Autodesk Inventor part; units mm, degrees
ref_plane "YZ Plane" through (0, 0, 0) normal (1, 0, 0) x (0, 1, 0)
ref_plane "XZ Plane" through (0, 0, 0) normal (0, 1, 0) x (-1, 0, 0)
ref_plane "XY Plane" through (0, 0, 0) normal (0, 0, 1) x (1, 0, 0)
sketch "Sketch1" plane through (0, 0, 0) normal (0, 0, 1) x (1, 0, 0)
  circle A0 centre (0, 0) radius 1.5
  circle A1 centre (0, 0) radius 3.5
  circle A2 centre (0, 0) radius 5.75 construction
  line L0 (0, 0) -> (0, 5.75) construction
  circle A3 centre (0.5, 9.2365) radius 3.5
  line L1 (0, 0) -> (0, 5.75) construction
  line L2 (3.5, 0) -> (3.5, 5.75)
  line L3 (-3.5, 5.75) -> (-3.5, 0)
  arc A4 (-3.5, 0) -> (3.5, 0) centre (0, 0) ccw
  arc A5 (3.5, 5.75) -> (-1.9961, 2.875) centre (0, 5.75) ccw
  arc A6 (-3.4062, 0.805) -> (-3.4062, 4.945) centre (-12.1649, 2.875) ccw
  line L4 (0.5, 5.7365) -> (3.5, 5.7365)
  point P0 (0, 2.875)
  point P1 (-3.4345, 6.424)
  point P2 (3.5, 0)
  point P3 (3.244, 7.0639)
  point P4 (-3.5, 0)
  point P5 (-2.744, 7.9226)
  dimension "d2" = 11.5
  dimension "d3" = 7
  dimension "d0" = 3
  dimension "d1" = 7
  dimension "d4" = 3.5
  dimension "d9" = 0.5
  dimension "d10" = 9
extrude "Extrusion1" add sketch "Sketch1" along normal blind 4.7625 contours A1 | A1 A5 A3 L4 L2 | A1 A6 A5 | L3 A5 A6 A1
fillet "Fillet1" radius 1 1 edges at (-2.744, 7.9226, 2.3813)
fillet "Fillet2" radius 1 1 edges at (3.5, 5.7365, 2.3813)
sketch "Sketch2" plane through (0, 0, 0) normal (0, 0, -1) x (-1, 0, 0)
  line L0 (-3.5, 0) -> (-3.5, 4.7365)
  arc A0 (-3.5, 0) -> (3.5, 0) centre (0, 0) ccw
  circle A1 centre (0, 0) radius 1.5
  circle A2 centre (0, 0) radius 6.3558 construction
  arc A3 (3.4953, 5.9311) -> (1.8307, 6.6254) centre (2.4966, 5.8794) ccw
  arc A4 (-0.5, 5.7365) -> (1.8307, 6.6254) centre (-0.5, 9.2365) ccw
  line L1 (3.5, 5.75) -> (3.5, 0)
  line L2 (-2.5, 5.7365) -> (-0.5, 5.7365)
  arc A5 (-2.5, 5.7365) -> (-3.5, 4.7365) centre (-2.5, 4.7365) ccw
  arc A6 (-2.5, 5.7365) -> (-3.5, 4.7365) centre (-2.5, 4.7365) ccw
  arc A7 (3.5, 5.75) -> (3.4953, 5.9311) centre (0, 5.75) ccw
equation "\"d4\" = 0.5 * d1"
properties part number "Cam - Lever" material "Nylon 6/6"
Work out the finished part from the listing and answer in its coordinate system (mm). Give positions to 0.01 mm unless a question says otherwise; leave off trailing zeros. Order: outer loops, then holes, each group sorted by start corner. A loop starts at its lowest first (then second) coordinate and runs counter-clockwise, first axis right, second up.
1. Section B-B, the plane x = -0.5 is taken. Determine the outline of the cut face in (y, z).
Result sheet:
outline: (-3.46, 0) - (-1.41, 0) - (-1.41, 4.76) - (-3.46, 4.76) - close; (1.41, 0) - (5.88, 0) - (5.88, 4.76) - (1.41, 4.76) - close
2. Straight lines are drawn through the part: L1, parallel to Y at x = -0.5, z = 2.1; L2, parallel to Y at x = 1.25, z = 3.85; L3, parallel to X at y = 1.25, z = 3.8. For each, find the intervals that lie inside material, in ascending order.
Result sheet:
L1: y = -3.46 to -1.41, 1.41 to 5.88
L2: y = -3.27 to -0.83, 0.83 to 5.74
L3: x = -3.5 to -0.83, 0.83 to 3.5
3. Section C-C, the plane y = -2.25 is taken. Determine the outline of the cut face in (x, z).
Result sheet:
outline: (-2.68, 0) - (2.68, 0) - (2.68, 4.76) - (-2.68, 4.76) - close
4. This flat-tipped pin is pushed along its axis until it touches: P1, Ø2, axis at x = 1.5, z = 1.5, coming from the +Y side. Where does it stop, or does it pass through?
Result sheet:
P1: stops at y = 5.74
5. The mould has two halves that part along Y. Classify faces 1 (the flat face through (0, 2, 0)), 2 (the cylindrical face through (-1.5, -0.07, 2.35)), 3 (the cylindrical face through (0.1, -3.5, 2.3)), 4 (the flat face through (1, 5.736, 2)): released by +Y, released by -Y, zero draft, split by the parting line, or undercut.
Result sheet:
face 1: zero draft
face 2: undercut
face 3: released by -Y
face 4: released by +Y
6. Section A-A, the plane y = 1 is taken. Determine the outline of the cut face in (x, z), and give its area (3 significant figures).
Result sheet:
outline: (-3.5, 0) - (-1.12, 0) - (-1.12, 4.76) - (-3.5, 4.76) - close; (1.12, 0) - (3.5, 0) - (3.5, 4.76) - (1.12, 4.76) - close
area: 22.7 mm2
